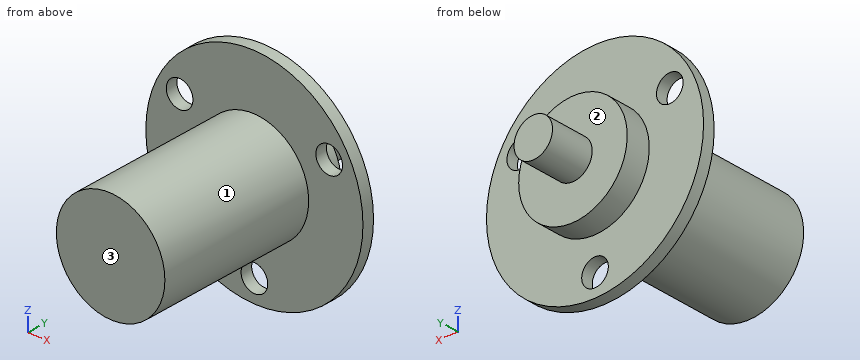
Autodesk Inventor part; units mm, degrees
ref_plane "YZ Plane" through (0, 0, 0) normal (1, 0, 0) x (0, 1, 0)
ref_plane "XZ Plane" through (0, 0, 0) normal (0, 1, 0) x (-1, 0, 0)
ref_plane "XY Plane" through (0, 0, 0) normal (0, 0, 1) x (1, 0, 0)
sketch "Sketch1" plane through (0, 0, 0) normal (0, 1, 0) x (-1, 0, 0)
  circle A0 centre (0, 0) radius 3.9
  dimension "d0" = 7.8
extrude "Extrusion1" add sketch "Sketch1" along normal blind 9
sketch "Sketch2" plane through (0, 0, 0) normal (0, -1, 0) x (1, 0, 0)
  circle A0 centre (0, 0) radius 11
  dimension "d3" = 22
extrude "Extrusion2" add sketch "Sketch2" along normal blind 5
sketch "Sketch3" plane through (0, -5, 0) normal (0, -1, 0) x (1, 0, 0)
  circle A0 centre (0, 0) radius 3.9
  circle A1 centre (0, 0) radius 22
  dimension "d6" = 44
extrude "Extrusion3" add sketch "Sketch3" along normal blind 2.4 contours A0 | A1
sketch "Sketch4" plane through (0, -7.4, 0) normal (0, -1, 0) x (1, 0, 0)
  circle A0 centre (0, 0) radius 11
  dimension "d9" = 22
extrude "Extrusion4" add sketch "Sketch4" along normal blind 32.6
sketch "Sketch6" plane through (0, -5, 0) normal (0, 1, 0) x (1, 0, 0)
  circle A0 centre (0, 0) radius 22
  circle A1 centre (0, 0) radius 11
  circle A2 centre (0, 0) radius 17.5
  circle A3 centre (0, 17.5) radius 2.7
  circle A4 centre (-15.1554, -8.75) radius 2.7
  circle A5 centre (15.1554, -8.75) radius 2.7
  dimension "d12" = 35
  dimension "d13" = 5.4
  dimension "d16" = 360
extrude "Extrusion5" cut sketch "Sketch6" against normal blind 27.6 contours A3 A2 | A2 A3 | A5 A2 | A2 A5 | A4 A2 | A2 A4
properties part number "Slip_ring"
Geometry check sheet. Reference: the model listing, model coordinates, mm. Face numbers are marked on the shaded views. A direction names the side the tool comes from. Coordinates: 2 decimals unless noted, no trailing zeros. Order: outer loops, then holes, each group sorted by start corner. A loop starts at its lowest first (then second) coordinate and runs counter-clockwise, first axis right, second up. Notation, with made-up numbers: (-16.5, -22) - (-9.5, -22) arc R4 cw to (-9.5, -16) - close; hole circle Ø2 at (-37.75, -11). An arc over 180 degrees is marked (long way). Answer in a Markdown table with one row per item. Add a question column.
1. Section check C-C (z = 0). Enter the section's corners in (x, y), plus the area to 3 significant figures.
2. Section check B-B (z = 8.75). Enter the section's corners in (x, y), plus the area to 3 significant figures.
3. Access from +Z, -Z, +X, -X, +Y, -Y to the whole of each face (thin tool, end or side, straight path). Record for the marked faces 1, 2 and 3.
4. Gauge pin test, flat ends, axial feed: pin 1 Ø8.5 at (x, z) = (15.16, 8.75) entering from +Y; pin 2 Ø7 at (x, z) = (-15.16, 8.75) entering from -Y; pin 3 Ø1.5 at (y, z) = (-9, -5.5) entering from +X; pin 4 Ø1 at (x, y) = (12, -13) entering from +Z. Record the tip position at first contact, or that the pin passes through.
5. Material ranges on L1, parallel to X at y = -6.2, z = 8.75; L2, parallel to Y at x = 18.5, z = 11; L3, parallel to X at y = -6.4, z = -17.5, recorded low to high. Write a range as [from, to].
6. Section check A-A (x = 0). Enter the section's corners in (y, z).
7. Section check D-D (y = -6.5). Enter the section's corners in (x, z).
Data:
| question | item | result |
|---|---|---|
| 1 | outline | (-22, -7.4) - (-11, -7.4) - (-11, -40) - (11, -40) - (11, -7.4) - (22, -7.4) - (22, -5) - (11, -5) - (11, 0) - (3.9, 0) - (3.9, 9) - (-3.9, 9) - (-3.9, 0) - (-11, 0) - (-11, -5) - (-22, -5) - close |
| 1 | area | 1,000 mm² |
| 2 | outline | (-20.19, -7.4) - (-17.86, -7.4) - (-17.86, -5) - (-20.19, -5) - close; (-12.46, -7.4) - (-6.67, -7.4) - (-6.67, -40) - (6.67, -40) - (6.67, -7.4) - (12.46, -7.4) - (12.46, -5) - (6.67, -5) - (6.67, 0) - (-6.67, 0) - (-6.67, -5) - (-12.46, -5) - close; (17.86, -7.4) - (20.19, -7.4) - (20.19, -5) - (17.86, -5) - close |
| 2 | area | 572 mm² |
| 3 | face 1 | -Y |
| 3 | face 2 | +Y |
| 3 | face 3 | +Z, -Z, +X, -X, -Y |
| 4 | pin 1 | stops at y = -5 |
| 4 | pin 2 | stops at y = -7.4 |
| 4 | pin 3 | stops at x = 9.92 |
| 4 | pin 4 | passes through |
| 5 | L1 | x = [-20.19, -17.86], [-12.46, 12.46], [17.86, 20.19] |
| 5 | L2 | y = [-7.4, -5] |
| 5 | L3 | x = [-13.33, -2.7], [2.7, 13.33] |
| 6 | outline | (-40, -11) - (-7.4, -11) - (-7.4, -14.8) - (-5, -14.8) - (-5, -11) - (0, -11) - (0, -3.9) - (9, -3.9) - (9, 3.9) - (0, 3.9) - (0, 11) - (-5, 11) - (-5, 22) - (-7.4, 22) - (-7.4, 11) - (-40, 11) - close; (-7.4, -22) - (-5, -22) - (-5, -20.2) - (-7.4, -20.2) - close |
| 7 | outline | circle Ø44 at (0, 0); hole circle Ø5.4 at (-15.16, 8.75); hole circle Ø5.4 at (0, -17.5); hole circle Ø5.4 at (15.16, 8.75) |
